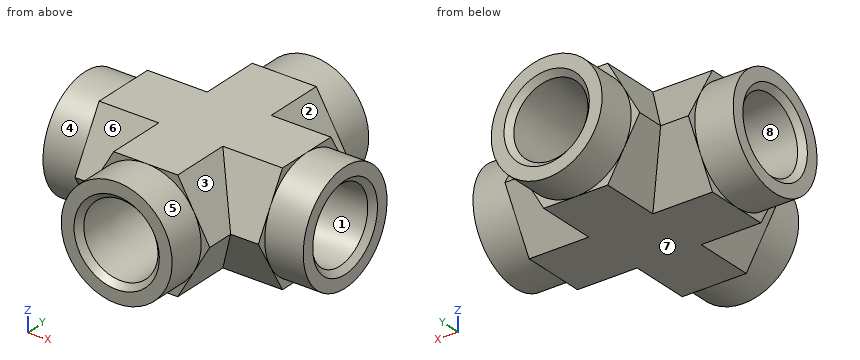
```python
from build123d import *
from OCP.BRepFilletAPI import BRepFilletAPI_MakeChamfer

# Parameters (mm, degrees)
BOSS_EXTRUDE1_START     = -21.997045256
BOSS_EXTRUDE1_DEPTH     = 26.746522628
BOSS_EXTRUDE1_START_2   = -16.497783942
BOSS_EXTRUDE1_2_DEPTH   = 10.998522628
BOSS_EXTRUDE1_START_3   = -10.998522628
BOSS_EXTRUDE1_3_DEPTH   = 21.997045256
BOSS_EXTRUDE2_DEPTH     = 4.749477372
BOSS_EXTRUDE3_DEPTH     = 4.749477372
BOSS_EXTRUDE4_DEPTH     = 4.749477372
SKETCH5_R               = 9.525
BOSS_EXTRUDE5_DEPTH     = 6.604
SKETCH10_R              = 6.402403746
CUT_EXTRUDE2_DEPTH      = 14.224
CUT_EXTRUDE2_DRAFT      = -1.788167188
CUT_EXTRUDE3_REACH      = 32.146
CUT_EXTRUDE3_END_RADIUS = 5.5499
SKETCH11_R              = 5.5499
SKETCH12_W              = 6.604
SKETCH12_H              = 9.525
SKETCH13_W              = 9.525
SKETCH13_H              = 6.604
SKETCH14_W              = 9.525
SKETCH14_H              = 6.604
CHAMFER1_SIZE           = 0.9271
CHAMFER1_SIZE2          = 0.957442613


with BuildPart() as part:
    # Boss-Extrude1: read off the stored shape, not the designer's step
    # Boss-Extrude1 outline → Boss-Extrude1 (new body)
    with BuildSketch(Plane.ZY.offset(10.998522628).offset(BOSS_EXTRUDE1_START)):
        Polygon((-9.525, 5.499261314), (-9.525, -5.499261314), (0, -10.998522628), (9.525, -5.499261314), (9.525, 5.499261314), (0, 10.998522628), align=None)
    extrude(amount=BOSS_EXTRUDE1_DEPTH)

    # Boss-Extrude1 2 outline → Boss-Extrude1 2 (add)
    with BuildSketch(Plane.ZY.offset(10.998522628).offset(BOSS_EXTRUDE1_START_2)):
        Polygon((-9.525, -5.499261314), (-9.525, -10.998522628), (0, -10.998522628), align=None)
        Polygon((9.525, -5.499261314), (0, -10.998522628), (9.525, -10.998522628), align=None)
        Polygon((-9.525, 10.998522628), (-9.525, 5.499261314), (0, 10.998522628), align=None)
        Polygon((9.525, 10.998522628), (0, 10.998522628), (9.525, 5.499261314), align=None)
    extrude(amount=BOSS_EXTRUDE1_2_DEPTH)

    # Boss-Extrude1 3 outline → Boss-Extrude1 3 (add)
    with BuildSketch(Plane(origin=(0, 0, 0), x_dir=(1, 0, 0), z_dir=(0, 1, 0)).offset(BOSS_EXTRUDE1_START_3)):
        Polygon((10.998522628, 0), (5.499261314, 9.525), (5.499261314, -9.525), align=None)
        Polygon((-10.998522628, 0), (-5.499261314, -9.525), (-5.499261314, 9.525), align=None)
    extrude(amount=BOSS_EXTRUDE1_3_DEPTH)

    # Sketch2 → Boss-Extrude2 (add)
    with BuildSketch(Plane.XZ.offset(10.998522628)):
        Polygon((-5.499261314, -9.525), (-10.998522628, 0), (-5.499261314, 9.525), (5.499261314, 9.525), (10.998522628, 0), (5.499261314, -9.525), align=None)
    extrude(amount=BOSS_EXTRUDE2_DEPTH)

    # Sketch3 → Boss-Extrude3 (add)
    with BuildSketch(Plane(origin=(0, 10.998522628, 0), x_dir=(-1, 0, 0), z_dir=(0, 1, 0))):
        Polygon((-5.499261314, 9.525), (5.499261314, 9.525), (10.998522628, 0), (5.499261314, -9.525), (-5.499261314, -9.525), (-10.998522628, 0), align=None)
    extrude(amount=BOSS_EXTRUDE3_DEPTH)

    # Sketch4 → Boss-Extrude4 (add)
    with BuildSketch(Plane(origin=(10.998522628, 0, 0), x_dir=(0, 0, -1), z_dir=(1, 0, 0))):
        Polygon((0, 10.998522628), (9.525, 5.499261314), (9.525, -5.499261314), (0, -10.998522628), (-9.525, -5.499261314), (-9.525, 5.499261314), align=None)
    extrude(amount=BOSS_EXTRUDE4_DEPTH)

    # Sketch5 → Boss-Extrude5 (add)
    with BuildSketch(Plane(origin=(15.748, 0, 0), x_dir=(0, 0, -1), z_dir=(1, 0, 0))):
        Circle(SKETCH5_R)
    extrude(amount=BOSS_EXTRUDE5_DEPTH)


with BuildPart() as cut_extrude2_tool:
    # Sketch10 → Cut-Extrude2 (with draft: the straight prism first)
    with BuildSketch(Plane(origin=(22.352, 0, 0), x_dir=(0, 0, -1), z_dir=(1, 0, 0))):
        Circle(SKETCH10_R)
    extrude(amount=-CUT_EXTRUDE2_DEPTH)
    # Cut-Extrude2: the draft: its side faces are tilted about the plane it starts from
    cut_extrude2_sides = [cut_extrude2_tool.faces().sort_by_distance(p)[0] for p in [
        (15.24, 0, 6.402403746),
    ]]
    draft(cut_extrude2_sides, Plane(origin=(22.352, 0, 0), x_dir=(0, 0, -1), z_dir=(1, 0, 0)), CUT_EXTRUDE2_DRAFT)


with BuildPart() as part_1:
    add(part.part)

    # Cut-Extrude2: cut by cut_extrude2_tool
    add(cut_extrude2_tool.part, mode=Mode.SUBTRACT)

    # Cut-Extrude3: up to this cylinder (the profile starts outside it)
    cut_extrude3_end = Plane(origin=(0, 0, 0), z_dir=(0, 1, 0)) * Cylinder(CUT_EXTRUDE3_END_RADIUS, 76.3918, mode=Mode.PRIVATE)
    # Sketch11 → Cut-Extrude3 (cut, up to the surface)
    with BuildSketch(Plane(origin=(8.128, 0, 0), x_dir=(0, 0, -1), z_dir=(1, 0, 0)), mode=Mode.PRIVATE) as cut_extrude3_sk1:
        with Locations(Location((0, 0, 0), (0, 0, 180))):
            Circle(SKETCH11_R)
    cut_extrude3_tool1 = extrude(cut_extrude3_sk1.sketch, amount=-CUT_EXTRUDE3_REACH, mode=Mode.PRIVATE) - cut_extrude3_end
    add(cut_extrude3_tool1.solids().sort_by_distance((8.128, 0, 0))[0], mode=Mode.SUBTRACT)

    # Sketch12 → Revolve1 (revolve)
    with BuildSketch(Plane(origin=(0, 0, 0), x_dir=(-1, 0, 0), z_dir=(0, 0, -1)), mode=Mode.PRIVATE) as revolve1_sk:
        with Locations((19.05, 4.7625)):
            Rectangle(SKETCH12_W, SKETCH12_H)
    revolve(revolve1_sk.sketch.rotate(Axis((-15.748, 0, 0), (-1, 0, 0)), 270), axis=Axis((-15.748, 0, 0), (-1, 0, 0)))

    # Sketch13 → Revolve2 (revolve)
    with BuildSketch(Plane.XY, mode=Mode.PRIVATE) as revolve2_sk:
        with Locations((4.7625, -19.05)):
            Rectangle(SKETCH13_W, SKETCH13_H)
    revolve(revolve2_sk.sketch.rotate(Axis((0, -15.748, 0), (0, -1, 0)), 270), axis=Axis((0, -15.748, 0), (0, -1, 0)))

    # Sketch14 → Revolve3 (revolve)
    with BuildSketch(Plane(origin=(0, 0, 0), x_dir=(-1, 0, 0), z_dir=(0, 0, -1)), mode=Mode.PRIVATE) as revolve3_sk:
        with Locations((-4.7625, 19.05)):
            Rectangle(SKETCH14_W, SKETCH14_H)
    revolve(revolve3_sk.sketch.rotate(Axis((0, 15.748, 0), (0, 1, 0)), 270), axis=Axis((0, 15.748, 0), (0, 1, 0)))

    # Sketch15 → Cut-Revolve1 (revolve, cut)
    with BuildSketch(Plane(origin=(0, 0, 0), x_dir=(-1, 0, 0), z_dir=(0, 0, -1)), mode=Mode.PRIVATE) as cut_revolve1_sk:
        Polygon((-6.402403746, -22.352), (0, -22.352), (0, 0), (-5.5499, 0), (-5.5499, -8.128), (-5.958336981, -8.128), align=None)
    revolve(cut_revolve1_sk.sketch.rotate(Axis((0, -22.352, 0), (0, 1, 0)), 270), axis=Axis((0, -22.352, 0), (0, 1, 0)), mode=Mode.SUBTRACT)

    # Sketch16 → Cut-Revolve2 (revolve, cut)
    with BuildSketch(Plane.XY, mode=Mode.PRIVATE) as cut_revolve2_sk:
        Polygon((6.402403746, 22.352), (0, 22.352), (0, 0), (5.5499, 0), (5.5499, 8.128), (5.958336981, 8.128), align=None)
    revolve(cut_revolve2_sk.sketch.rotate(Axis((0, 22.352, 0), (0, -1, 0)), 90), axis=Axis((0, 22.352, 0), (0, -1, 0)), mode=Mode.SUBTRACT)

    # Sketch17 → Cut-Revolve3 (revolve, cut)
    with BuildSketch(Plane.XY, mode=Mode.PRIVATE) as cut_revolve3_sk:
        Polygon((-22.352, 6.402403746), (-22.352, 0), (0, 0), (0, 5.5499), (-8.128, 5.5499), (-8.128, 5.958336981), align=None)
    revolve(cut_revolve3_sk.sketch.rotate(Axis((-22.352, 0, 0), (1, 0, 0)), 270), axis=Axis((-22.352, 0, 0), (1, 0, 0)), mode=Mode.SUBTRACT)

    # Chamfer1: one chamfer whose edges measure the first distance from different faces: ONE call of the kernel's chamfer builder (chamfer() names one face for all edges)
    chamfer1_edges_1 = [part_1.edges().sort_by_distance(p)[0] for p in [
        (22.352, 0, 6.402403746),
    ]]
    chamfer1_side_1 = [part_1.faces().sort_by_distance(p)[0] for p in [
        (15.24, 0, 6.180370364),
    ]]
    chamfer1_edges_2 = [part_1.edges().sort_by_distance(p)[0] for p in [
        (0, -22.352, -6.402403746),
    ]]
    chamfer1_side_2 = [part_1.faces().sort_by_distance(p)[0] for p in [
        (0, -22.352, 9.255592316),
    ]]
    chamfer1_edges_3 = [part_1.edges().sort_by_distance(p)[0] for p in [
        (0, 22.352, -6.402403746),
    ]]
    chamfer1_side_3 = [part_1.faces().sort_by_distance(p)[0] for p in [
        (0, 22.352, -9.255592316),
    ]]
    chamfer1_edges_4 = [part_1.edges().sort_by_distance(p)[0] for p in [
        (-22.352, 0, 6.402403746),
    ]]
    chamfer1_side_4 = [part_1.faces().sort_by_distance(p)[0] for p in [
        (-22.352, 0, -9.255592316),
    ]]
    chamfer1 = BRepFilletAPI_MakeChamfer(part_1.part.solid().wrapped)
    for e in chamfer1_edges_1:
        chamfer1.Add(CHAMFER1_SIZE, CHAMFER1_SIZE2, e.wrapped, chamfer1_side_1[0].wrapped)  # the first distance lies on this face
    for e in chamfer1_edges_2:
        chamfer1.Add(CHAMFER1_SIZE, CHAMFER1_SIZE2, e.wrapped, chamfer1_side_2[0].wrapped)  # the first distance lies on this face
    for e in chamfer1_edges_3:
        chamfer1.Add(CHAMFER1_SIZE, CHAMFER1_SIZE2, e.wrapped, chamfer1_side_3[0].wrapped)  # the first distance lies on this face
    for e in chamfer1_edges_4:
        chamfer1.Add(CHAMFER1_SIZE, CHAMFER1_SIZE2, e.wrapped, chamfer1_side_4[0].wrapped)  # the first distance lies on this face
    add(Compound.cast(chamfer1.Shape()), mode=Mode.REPLACE)


solid = part_1.part
```
Model file for the job. Use its own axes, mm. Face numbers are marked on the shaded views. A direction names the side the tool comes from. Coordinates: 2 decimals unless noted, no trailing zeros. Write each loop counter-clockwise with the first axis right and the second up, starting at its lowest first coordinate (ties: lowest second). Pieces come first, ordered by that corner, then holes. Notation, with made-up numbers: (-35, -5) - (0, -5) arc R18 cw to (0, 25) - close; hole circle Ø6 at (61, -40). An arc over 180 degrees is marked (long way). One line per question, with ' | ' between items. Start each with the question number.
Q1. 3-axis set-ups, long thin cutter, end or side, ignore diameter. For the marked faces 1, 2, 3 and 4: which of +Z, -Z, +X, -X, +Y, -Y reach the whole face in a straight line?
Q2. Cut at B-B, the plane z = 8. List the corners of the cut face in (x, y), then the cut area to 3 significant figures.
Q3. Pin check, flat tips, straight feed: pin 1 (5 mm diameter, centred on y = 14.5, z = 2, fed in from +X); pin 2 (1.5 mm diameter, centred on y = -5, z = -3, fed in from +X); pin 3 (2 mm diameter, centred on y = -13.5, z = -3, fed in from -X). Stop position of each tip, or through.
Q4. Drill centre lines: line 1 (Z direction, x = 0, y = 3) (3 decimals); line 2 (X direction, y = -5.75, z = 0); line 3 (Y direction, x = -8, z = 8). Where is each one in solid material? Low to high. Write a range as [from, to].
Q5. Pull direction Z, two halves, no side cores. Call the marked faces 5, 6, 7 and 8: pulls with the +Z half, pulls with the -Z half, needs draft (parallel to the pull), parting line crosses it, or undercut.
Q6. Cut at C-C, the plane z = 2.5. Give the number of separate pieces and of enclosed holes in the cut face, then the cut area to 3 significant figures.
Q7. Cut at A-A, the plane y = -14.5. List the corners of the cut face in (x, z) (3 decimals).
Answer below:
1) face 1: +X | face 2: +Z, +X, +Y | face 3: +Z, +X, -Y | face 4: -X
2) outline: (-22.35, -5.17) - (-15.75, -5.17) - (-15.75, -6.38) - (-6.38, -6.38) - (-6.38, -15.75) - (-5.17, -15.75) - (-5.17, -22.35) - (5.17, -22.35) - (5.17, -15.75) - (6.38, -15.75) - (6.38, -6.38) - (15.75, -6.38) - (15.75, -5.17) - (22.35, -5.17) - (22.35, 5.17) - (15.75, 5.17) - (15.75, 6.38) - (6.38, 6.38) - (6.38, 15.75) - (5.17, 15.75) - (5.17, 22.35) - (-5.17, 22.35) - (-5.17, 15.75) - (-6.38, 15.75) - (-6.38, 6.38) - (-15.75, 6.38) - (-15.75, 5.17) - (-22.35, 5.17) - close | area: 914 mm^2
3) pin 1: x = 11 | pin 2: x = 21.62 | pin 3: x = -9.84
4) line 1: [-9.525, -5.55], [5.55, 9.525] | line 2: [-8.13, -5.55], [5.55, 8.13] | line 3: [-6.38, 6.38]
5) face 5: parting line crosses it | face 6: pulls with the +Z half | face 7: pulls with the -Z half | face 8: undercut
6) separate pieces: 4 | enclosed holes: 0 | area: 453 mm^2
7) outline: (-10.999, 0) - (-5.499, -9.525) - (5.499, -9.525) - (10.999, 0) - (5.499, 9.525) - (-5.499, 9.525) - close; hole circle Ø12.315 at (0, 0)
